Read the model definition and answer for the solid it produces. Units are mm, in the model's axes. Give positions to 0.01 mm unless a question says otherwise; leave off trailing zeros. Order: outer loops, then holes, each group sorted by start corner. A loop starts at its lowest first (then second) coordinate and runs counter-clockwise, first axis right, second up. Notation, with made-up numbers: (42, 82.5) - (62, 82.5) arc R13 ccw to (62, 89.5) - close; hole circle Ø8 at (9, 75.5). An arc over 180 degrees is marked (long way). Write each question's results on one line, items separated by ' | '.
from build123d import *

# Parameters (mm, degrees)
SKETCH1_R           = 1.5875
SKETCH1_R_2         = 0.8763
BOSS_EXTRUDE1_DEPTH = 282.575
SKETCH3_R           = 0.396875
CUT_EXTRUDE1_DEPTH  = 2.159
CHAMFER1_SIZE       = 0.762


with BuildPart() as part:
    # Sketch1 → Boss-Extrude1 (new body)
    with BuildSketch(Plane.XY):
        Circle(SKETCH1_R)
        Circle(SKETCH1_R_2, mode=Mode.SUBTRACT)
    extrude(amount=BOSS_EXTRUDE1_DEPTH)

    # Sketch3 → Cut-Extrude1 (cut, symmetric)
    with BuildSketch(Plane(origin=(0, 0, 0), x_dir=(0, 0, -1), z_dir=(1, 0, 0))):
        with Locations((-279.9969, 0)):
            Circle(SKETCH3_R)
        with Locations((-275.082, 0)):
            Circle(SKETCH3_R)
    extrude(amount=CUT_EXTRUDE1_DEPTH, both=True, mode=Mode.SUBTRACT)

    # Chamfer1
    # the kernel refuses this chamfer: 0.762 mm, written as the material it takes off along each edge
    with BuildSketch(Plane(origin=(0, 0, 0), x_dir=(1, 0, 0), z_dir=(0, -1, 0))) as chamfer1_piece_1:
        Polygon((1.5875, CHAMFER1_SIZE), (1.5875 - CHAMFER1_SIZE, 0), (1.5875, 0), align=None)
    revolve(axis=Axis((0, 0, 0), (0, 0, 1)), mode=Mode.SUBTRACT)


solid = part.part
(1) Section B-B (z = 258) is taken. Give the vertices of the cut face in (x, y) (1 decimal), plus the area to 3 significant figures.
Conclusion:
outline: circle Ø3.2 at (0, 0); hole circle Ø1.8 at (0, 0) | area: 5.50 mm^2
(2) Consider probe 1 along X at (y, z) = (0.2, 186); probe 2 along X at (y, z) = (0.3, 125.5). Determine where each line is inside the solid, lowest interval first. Write a range as [from, to].
Conclusion:
probe 1: [-1.57, -0.85], [0.85, 1.57] | probe 2: [-1.56, -0.82], [0.82, 1.56]
(3) This flat-tipped pin is pushed along its axis until it touches: pin 1 (1.4 mm diameter, centred on x = 0, y = 0, fed in from -Z). Where does it stop, or does it pass through?
Conclusion:
pin 1: through
(4) Section A-A (x = 0) is taken. Give the vertices of the cut face in (y, z) (1 decimal).
Conclusion:
outline: (-1.6, 0.8) - (-0.9, 0.1) - (-0.9, 282.6) - (-1.6, 282.6) - close; (0.9, 0.1) - (1.6, 0.8) - (1.6, 282.6) - (0.9, 282.6) - close
